Design review of the part built by this model. Coordinates are the model's own, in mm. Face numbers are marked on the shaded views. A direction names the side the tool comes from. Round coordinates to 2 decimals unless told otherwise and drop trailing zeros. Loops run counter-clockwise (first coordinate to the right, second up) from the corner with the lowest first, then second, coordinate; pieces in that order, holes last. Notation, with made-up numbers: (-0.75, 62.5) - (7.25, 62.5) arc R21 cw to (7.25, 70.5) - close; hole circle Ø7 at (22, 87.5). An arc over 180 degrees is marked (long way). Answer as CSV lines item,"result". Start each with the question number.
(1) Mouldability with a two-part tool opening along X and no side actions: class the marked faces 6, 7 and 8 as released by +X, released by -X, zero draft, split by the parting line, or undercut.
(2) For P1, Ø1.8, axis at x = -16, y = 11.5, coming from the +Z side; P2, Ø10, axis at x = -153.5, z = -34, coming from the +Y side; P3, Ø8, axis at x = -97.5, y = 58.5, coming from the -Z side; P4, Ø5, axis at x = 4, z = -24, coming from the -Y side, all flat-tipped, find the tip position at first contact; note any pin that passes through.
(3) For the marked faces 1, 2, 3, 4 and 5, list the 3-axis set-ups (+Z, -Z, +X, -X, +Y, -Y) from which the entire face can be reached by the end or side of a thin tool; tool diameter is ignored.
(4) Consider section A-A (x = 0). Give the boundary of the cut face in (y, z), and give its area (3 significant figures).
(5) Consider section B-B (y = 99). Give the boundary of the cut face in (x, z), and give its area (3 significant figures).
(6) Wall thickness on L1, parallel to Y at x = -63, z = 33.5; L2, parallel to Y at x = -128.5, z = -47.5; L3, parallel to X at y = 31.5, z = -3.5: over which ranges is each line inside the solid? List them lowest first.
from build123d import *

# Parameters (mm, degrees)
SKETCH1_R                    = 150
BOSS_EXTRUDE1_DEPTH          = 75
CHAMFER1_SIZE                = 10
BOSS_EXTRUDE2_START          = -75
SKETCH2_R                    = 150
BOSS_EXTRUDE2_DEPTH          = 10
CHAMFER2_SIZE                = 10
CHAMFER3_SIZE                = 10
BOSS_EXTRUDE3_DEPTH          = 9
BOSS_EXTRUDE4_DEPTH          = 3.5
CIRPATTERN1_COUNT            = 4
CIRPATTERN1_COPY_1_DEPTH     = 9
CIRPATTERN1_COPY_2_DEPTH     = 9
CIRPATTERN1_COPY_3_DEPTH     = 9
CIRPATTERN1_COPY_4_DEPTH     = 3.5
CIRPATTERN1_COPY_5_DEPTH     = 3.5
CIRPATTERN1_COPY_6_DEPTH     = 3.5
CHAMFER2_OF_CIRPATTERN1_SIZE = 10
CHAMFER3_OF_CIRPATTERN1_SIZE = 10
CUT_EXTRUDE1_START           = -60
CUT_EXTRUDE1_DEPTH           = 60
SKETCH7_R                    = 110
BOSS_EXTRUDE5_DEPTH          = 10
BOSS_EXTRUDE5_TAPER          = 45
SKETCH8_R                    = 15
BOSS_EXTRUDE6_DEPTH          = 20


with BuildPart() as part:
    # Sketch1 → Boss-Extrude1 (new body)
    with BuildSketch(Plane(origin=(0, 0, 0), x_dir=(1, 0, 0), z_dir=(0, 1, 0))):
        with Locations(Location((0, 0, 0), (0, 0, 270))):
            Circle(SKETCH1_R)
    extrude(amount=BOSS_EXTRUDE1_DEPTH)

    # Chamfer1
    chamfer1_edges = [part.edges().sort_by_distance(p)[0] for p in [
        (0, 75, -150),
    ]]
    chamfer(chamfer1_edges, length=CHAMFER1_SIZE)

    # Sketch2 → Boss-Extrude2 (add)
    with BuildSketch(Plane(origin=(0, 75, 0), x_dir=(1, 0, 0), z_dir=(0, 1, 0)).offset(BOSS_EXTRUDE2_START)):
        with Locations(Location((0, 0, 0), (0, 0, 165.522487814))):
            Circle(SKETCH2_R)
        with BuildLine():
            Line((-145.236875483, 37.5), (-195.236875483, 37.5))
            Line((-195.236875483, 37.5), (-195.236875483, -37.5))
            Line((-195.236875483, -37.5), (-145.236875483, -37.5))
            ThreePointArc((-145.236875483, -37.5), (-150, 0), (-145.236875483, 37.5))
        make_face()
    boss_extrude2 = extrude(amount=BOSS_EXTRUDE2_DEPTH)

    # Chamfer2
    chamfer2_edges = [part.edges().sort_by_distance(p)[0] for p in [
        (-195.236875483, 5, 37.5),
    ]]
    chamfer(chamfer2_edges, length=CHAMFER2_SIZE)

    # Chamfer3
    chamfer3_edges = [part.edges().sort_by_distance(p)[0] for p in [
        (-195.236875483, 5, -37.5),
    ]]
    chamfer(chamfer3_edges, length=CHAMFER3_SIZE)

    # Sketch3 → Boss-Extrude3 (add)
    with BuildSketch(Plane.XY.offset(37.5)):
        Polygon((-185.236875483, 10), (-145.236875483, 10), (-145.236875483, 65), (-170.236875483, 65), align=None)
    boss_extrude3 = extrude(amount=-BOSS_EXTRUDE3_DEPTH)

    # Sketch4 → Boss-Extrude4 (add)
    with BuildSketch(Plane(origin=(0, 10, 0), x_dir=(1, 0, 0), z_dir=(0, 1, 0))):
        Polygon((-180.04072306, -12), (-185.236875483, -9), (-190.433027905, -12), (-190.433027905, -18), (-185.236875483, -21), (-180.04072306, -18), align=None)
    boss_extrude4 = extrude(amount=BOSS_EXTRUDE4_DEPTH)

    # Mirror1: Boss-Extrude3, Boss-Extrude4 across plane
    add(boss_extrude3.mirror(Plane.XY))
    add(boss_extrude4.mirror(Plane.XY))

    # CirPattern1: Boss-Extrude2, Boss-Extrude3, Boss-Extrude4 ×4 about axis
    cirpattern1_axis = Axis((0, 0, 0), (0, 1, 0))
    add([boss_extrude2.rotate(cirpattern1_axis, i * 360 / CIRPATTERN1_COUNT) for i in range(1, CIRPATTERN1_COUNT)])
    add([boss_extrude3.rotate(cirpattern1_axis, i * 360 / CIRPATTERN1_COUNT) for i in range(1, CIRPATTERN1_COUNT)])
    add([boss_extrude4.rotate(cirpattern1_axis, i * 360 / CIRPATTERN1_COUNT) for i in range(1, CIRPATTERN1_COUNT)])

    # CirPattern1 copy 1 sketch → CirPattern1 copy 1 (add)
    with BuildSketch(Plane(origin=(-37.5, 0, 0), x_dir=(0, 0, -1), z_dir=(-1, 0, 0))):
        Polygon((-185.236875483, -10), (-145.236875483, -10), (-145.236875483, -65), (-170.236875483, -65), align=None)
    extrude(amount=-CIRPATTERN1_COPY_1_DEPTH)

    # CirPattern1 copy 2 sketch → CirPattern1 copy 2 (add)
    with BuildSketch(Plane(origin=(0, 0, 37.5), x_dir=(-1, 0, 0), z_dir=(0, 0, 1))):
        Polygon((-185.236875483, -10), (-145.236875483, -10), (-145.236875483, -65), (-170.236875483, -65), align=None)
    extrude(amount=-CIRPATTERN1_COPY_2_DEPTH)

    # CirPattern1 copy 3 sketch → CirPattern1 copy 3 (add)
    with BuildSketch(Plane(origin=(37.5, 0, 0), x_dir=(0, 0, 1), z_dir=(1, 0, 0))):
        Polygon((-185.236875483, -10), (-145.236875483, -10), (-145.236875483, -65), (-170.236875483, -65), align=None)
    extrude(amount=-CIRPATTERN1_COPY_3_DEPTH)

    # CirPattern1 copy 4 sketch → CirPattern1 copy 4 (add)
    with BuildSketch(Plane(origin=(0, 10, 0), x_dir=(0, 0, -1), z_dir=(0, 1, 0))):
        Polygon((-180.04072306, 12), (-185.236875483, 9), (-190.433027905, 12), (-190.433027905, 18), (-185.236875483, 21), (-180.04072306, 18), align=None)
    extrude(amount=CIRPATTERN1_COPY_4_DEPTH)

    # CirPattern1 copy 5 sketch → CirPattern1 copy 5 (add)
    with BuildSketch(Plane(origin=(0, 10, 0), x_dir=(-1, 0, 0), z_dir=(0, 1, 0))):
        Polygon((-180.04072306, 12), (-185.236875483, 9), (-190.433027905, 12), (-190.433027905, 18), (-185.236875483, 21), (-180.04072306, 18), align=None)
    extrude(amount=CIRPATTERN1_COPY_5_DEPTH)

    # CirPattern1 copy 6 sketch → CirPattern1 copy 6 (add)
    with BuildSketch(Plane.ZX.offset(10)):
        Polygon((-180.04072306, 12), (-185.236875483, 9), (-190.433027905, 12), (-190.433027905, 18), (-185.236875483, 21), (-180.04072306, 18), align=None)
    extrude(amount=CIRPATTERN1_COPY_6_DEPTH)

    # Chamfer2 of CirPattern1
    chamfer2_of_cirpattern1_edges = [part.edges().sort_by_distance(p)[0] for p in [
        (37.5, 5, 195.236875483),
        (195.236875483, 5, -37.5),
        (-37.5, 5, -195.236875483),
    ]]
    chamfer(chamfer2_of_cirpattern1_edges, length=CHAMFER2_OF_CIRPATTERN1_SIZE)

    # Chamfer3 of CirPattern1
    chamfer3_of_cirpattern1_edges = [part.edges().sort_by_distance(p)[0] for p in [
        (-37.5, 5, 195.236875483),
        (195.236875483, 5, 37.5),
        (37.5, 5, -195.236875483),
    ]]
    chamfer(chamfer3_of_cirpattern1_edges, length=CHAMFER3_OF_CIRPATTERN1_SIZE)

    # Sketch5 → Cut-Extrude1 (cut)
    with BuildSketch(Plane(origin=(0, 75, 0), x_dir=(1, 0, 0), z_dir=(0, 1, 0)).offset(CUT_EXTRUDE1_START)):
        with BuildLine():
            ThreePointArc((-70, -121.24355653), (-98.994949366, -98.994949366), (-121.24355653, -70))
            Line((-121.24355653, -70), (-129.903810568, -75))
            ThreePointArc((-129.903810568, -75), (-106.066017178, -106.066017178), (-75, -129.903810568))
            Line((-75, -129.903810568), (-70, -121.24355653))
        make_face()
        with BuildLine():
            ThreePointArc((-65, -112.583302492), (-91.923881554, -91.923881554), (-112.583302492, -65))
            Line((-112.583302492, -65), (-121.24355653, -70))
            ThreePointArc((-121.24355653, -70), (-98.994949366, -98.994949366), (-70, -121.24355653))
            Line((-70, -121.24355653), (-65, -112.583302492))
        make_face()
    extrude(amount=CUT_EXTRUDE1_DEPTH, mode=Mode.SUBTRACT)

    # Sketch7 → Boss-Extrude5 (add)
    with BuildSketch(Plane(origin=(0, 75, 0), x_dir=(1, 0, 0), z_dir=(0, 1, 0))):
        Circle(SKETCH7_R)
    extrude(amount=BOSS_EXTRUDE5_DEPTH, taper=BOSS_EXTRUDE5_TAPER)

    # Sketch8 → Boss-Extrude6 (add)
    with BuildSketch(Plane(origin=(0, 85, 0), x_dir=(1, 0, 0), z_dir=(0, 1, 0))):
        with Locations(Location((0, 0, 0), (0, 0, 270))):
            Circle(SKETCH8_R)
    extrude(amount=BOSS_EXTRUDE6_DEPTH)


solid = part.part
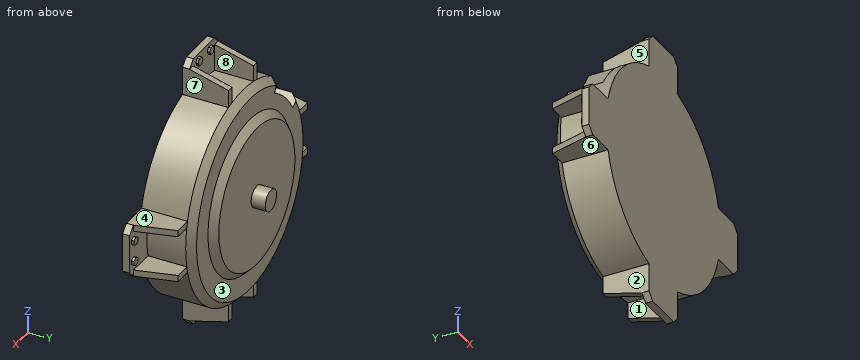
Determined:
1,face 6,"zero draft"
1,face 7,"released by +X"
1,face 8,"undercut"
2,P1,"stops at z = 190.43"
2,P2,"stops at y = 65"
2,P3,"stops at z = -117.29"
2,P4,"stops at y = 0"
3,face 1,"-Z, +Y"
3,face 2,"-Z, -X, +Y, -Y"
3,face 3,"+Y"
3,face 4,"+Z, +X, +Y, -Y"
3,face 5,"+Z, -X, +Y, -Y"
4,outline,"(0, -195.24) - (10, -195.24) - (10, -150) - (65, -150) - (75, -140) - (75, -110) - (85, -100) - (85, -15) - (105, -15) - (105, 15) - (85, 15) - (85, 100) - (75, 110) - (75, 140) - (65, 150) - (10, 150) - (10, 195.24) - (0, 195.24) - close"
4,area,"26,000 mm^2"
5,outline,"circle Ø30 at (0, 0)"
5,area,"707 mm^2"
6,L1,"y = 0 to 85"
6,L2,"y = 0 to 75"
6,L3,"x = -149.96 to 149.96"
